Design review of the part built by this model. Coordinates are the model's own, in mm. Coordinates: 2 decimals unless noted, no trailing zeros. Write each loop counter-clockwise with the first axis right and the second up, starting at its lowest first coordinate (ties: lowest second). Pieces come first, ordered by that corner, then holes. Notation, with made-up numbers: (83.25, 53) - (118.25, 53) arc R21 ccw to (118.25, 57) - close; hole circle Ø4 at (60.25, 56). An arc over 180 degrees is marked (long way). Answer as CSV lines item,"result". Start each with the question number.
Q1. We need section D-D (z = 0.95). Write out the cut boundary in (x, y), plus the area to 3 significant figures.
Q2. We need section C-C (y = -32.5). Write out the cut boundary in (x, z), plus the area to 3 significant figures.
Q3. For line 1 along Y through (x, z) = (6.25, 0.65); line 2 along Y through (x, z) = (0, 0.55); line 3 along Z through (x, y) = (8, -30), list the stretches that pass through material, from the lowest coordinate up. Write a range as [from, to].
Q4. Clearance check with a flat-ended pin moving along its axis: pin 1 (5.5 mm diameter, centred on x = -6.25, y = -32.5, fed in from -Z). State where the tip first meets the part, or that it passes through.
Q5. We need section B-B (x = 0). Write out the cut boundary in (y, z).
Q6. Mouldability with a two-part tool opening along X and no side actions: class faces 1 (the face through (12.5, -1, 1)), 2 (the face through (0, 36, 1)), 3 (the face through (-12.5, -1, 1)), 4 (the face through (0, 1, 3)) as pulls with the +X half, pulls with the -X half, needs draft (parallel to the pull), parting line crosses it, or undercut.
Q7. We need section A-A (y = 32.5). Write out the cut boundary in (x, z), plus the area to 3 significant figures.
from build123d import *

# Parameters (mm, degrees)
CROQUIS1_W              = 25
CROQUIS1_H              = 80
CROQUIS1_R              = 3.5
CROQUIS1_R_2            = 3.009292022
SALIENTE_EXTRUIR1_DEPTH = 3
REDONDEO1_R             = 0.5


with BuildPart() as part:
    # Croquis1 → Saliente-Extruir1 (new body)
    with BuildSketch(Plane.XY):
        Rectangle(CROQUIS1_W, CROQUIS1_H)
        with Locations((0, 32.5)):
            Circle(CROQUIS1_R, mode=Mode.SUBTRACT)
        with Locations((6.25, -32.5)):
            Circle(CROQUIS1_R_2, mode=Mode.SUBTRACT)
        with Locations(Location((-6.25, -32.5, 0), (0, 0, 180))):
            Circle(CROQUIS1_R_2, mode=Mode.SUBTRACT)
    extrude(amount=SALIENTE_EXTRUIR1_DEPTH)

    # Redondeo1
    redondeo1_edges = [part.edges().sort_by_distance(p)[0] for p in [
        (-3.5, 32.5, 3),
        (-12.5, 0, 3),
        (3.240707978, -32.5, 3),
        (0, -40, 3),
        (-3.240707978, -32.5, 3),
        (12.5, 0, 3),
        (0, -40, 0),
        (-12.5, 0, 0),
        (0, 40, 0),
        (12.5, 0, 0),
        (12.5, -40, 1.5),
        (-12.5, -40, 1.5),
        (-12.5, 40, 1.5),
        (12.5, 40, 1.5),
        (0, 40, 3),
    ]]
    fillet(redondeo1_edges, radius=REDONDEO1_R)


solid = part.part
Results list:
1,outline,"(-12.5, -39.5) arc R0.5 ccw to (-12, -40) - (12, -40) arc R0.5 ccw to (12.5, -39.5) - (12.5, 39.5) arc R0.5 ccw to (12, 40) - (-12, 40) arc R0.5 ccw to (-12.5, 39.5) - close; hole circle Ø6.02 at (-6.25, -32.5); hole circle Ø7 at (0, 32.5); hole circle Ø6.02 at (6.25, -32.5)"
1,area,"1,900 mm2"
2,outline,"(-12.5, 0.5) arc R0.5 ccw to (-12, 0) - (-9.26, 0) - (-9.26, 2.5) arc R0.5 ccw to (-9.76, 3) - (-12, 3) arc R0.5 ccw to (-12.5, 2.5) - close; (-3.24, 0) - (3.24, 0) - (3.24, 2.5) arc R0.5 ccw to (2.74, 3) - (-2.74, 3) arc R0.5 ccw to (-3.24, 2.5) - close; (9.26, 0) - (12, 0) arc R0.5 ccw to (12.5, 0.5) - (12.5, 2.5) arc R0.5 ccw to (12, 3) - (9.76, 3) arc R0.5 ccw to (9.26, 2.5) - close"
2,area,"38.5 mm2"
3,line 1,"y = [-40, -35.51], [-29.49, 40]"
3,line 2,"y = [-40, 29], [36, 40]"
3,line 3,"z = [0, 2.7]"
4,pin 1,"passes through"
5,outline,"(-40, 0.5) arc R0.5 ccw to (-39.5, 0) - (29, 0) - (29, 2.5) arc R0.5 ccw to (28.5, 3) - (-39.5, 3) arc R0.5 ccw to (-40, 2.5) - close; (36, 0) - (39.5, 0) arc R0.5 ccw to (40, 0.5) - (40, 2.5) arc R0.5 ccw to (39.5, 3) - (36.5, 3) arc R0.5 ccw to (36, 2.5) - close"
6,face 1,"pulls with the +X half"
6,face 2,"undercut"
6,face 3,"pulls with the -X half"
6,face 4,"needs draft"
7,outline,"(-12.5, 0.5) arc R0.5 ccw to (-12, 0) - (-3.5, 0) - (-3.5, 2.5) arc R0.5 ccw to (-4, 3) - (-12, 3) arc R0.5 ccw to (-12.5, 2.5) - close; (3.5, 0) - (12, 0) arc R0.5 ccw to (12.5, 0.5) - (12.5, 2.5) arc R0.5 ccw to (12, 3) - (4, 3) arc R0.5 ccw to (3.5, 2.5) - close"
7,area,"53.7 mm2"
